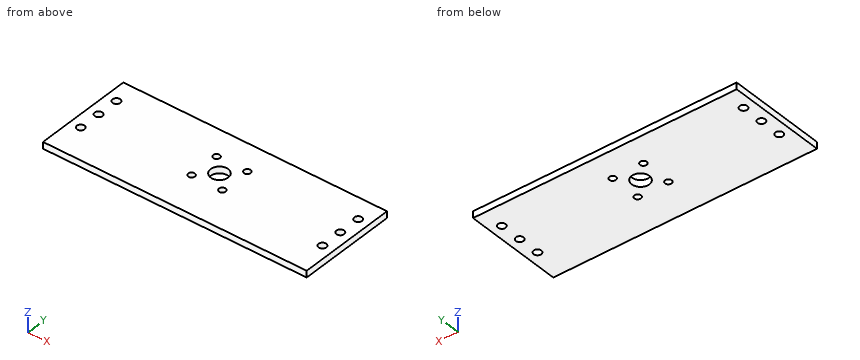
from build123d import *

# Parameters (mm, degrees)
ESQUISSE1_W             = 120
ESQUISSE1_H             = 45
BOSS_EXTRU_1_DEPTH      = 3
ESQUISSE2_R             = 1.747592995
ESQUISSE2_R_2           = 4
ESQUISSE2_R_3           = 1.5
ENL_V_MAT_EXTRU_1_DEPTH = 10


with BuildPart() as part:
    # Esquisse1 → Boss.-Extru.1 (new body)
    with BuildSketch(Plane.XY):
        Rectangle(ESQUISSE1_W, ESQUISSE1_H)
    extrude(amount=BOSS_EXTRU_1_DEPTH)

    # Esquisse2 → Enlèv. mat.-Extru.1 (cut)
    with BuildSketch(Plane.XY.offset(3)):
        with Locations((-55, 12.5)):
            Circle(ESQUISSE2_R)
        with Locations((55, 12.5)):
            Circle(ESQUISSE2_R)
        with Locations((-55, 2.5)):
            Circle(ESQUISSE2_R)
        with Locations((-55, -7.5)):
            Circle(ESQUISSE2_R)
        with Locations((55, -7.5)):
            Circle(ESQUISSE2_R)
        with Locations((55, 2.5)):
            Circle(ESQUISSE2_R)
        with Locations((0, 2.5)):
            Circle(ESQUISSE2_R_2)
        with Locations((-7, 9.5)):
            Circle(ESQUISSE2_R_3)
        with Locations((7, 9.5)):
            Circle(ESQUISSE2_R_3)
        with Locations((7, -4.5)):
            Circle(ESQUISSE2_R_3)
        with Locations((-7, -4.5)):
            Circle(ESQUISSE2_R_3)
    extrude(amount=-ENL_V_MAT_EXTRU_1_DEPTH, mode=Mode.SUBTRACT)


solid = part.part
Could you check a few things on this model? Use its own coordinates, in mm. Coordinates: 2 decimals unless noted, no trailing zeros. Write each loop counter-clockwise with the first axis right and the second up, starting at its lowest first coordinate (ties: lowest second). Pieces come first, ordered by that corner, then holes. Notation, with made-up numbers: (20.5, -12) - (33.5, -12) arc R30 cw to (33.5, 18) - close; hole circle Ø2 at (85, -33.5). An arc over 180 degrees is marked (long way). Write item = value, one per line.
1) Suppose I cut it at B-B on y = 2.5. Please give me the cut outline in (x, z), plus the area to 3 significant figures.
Result set:
outline = (-60, 0) - (-56.75, 0) - (-56.75, 3) - (-60, 3) - close; (-53.25, 0) - (-4, 0) - (-4, 3) - (-53.25, 3) - close; (4, 0) - (53.25, 0) - (53.25, 3) - (4, 3) - close; (56.75, 0) - (60, 0) - (60, 3) - (56.75, 3) - close
area = 315 mm2
2) Suppose I cut it at C-C on z = 1.6. State how many separate pieces and enclosed holes the cut face has, plus the area to 3 significant figures.
Result set:
separate_pieces = 1
enclosed_holes = 11
area = 5,260 mm2
3) Please list where these lines run through material, in increasing order: line 1 (Y direction, x = -55, z = 1.3); line 2 (Y direction, x = -7, z = 0.75); line 3 (X direction, y = 8.5, z = 1). Write a range as [from, to].
Result set:
line_1 = [-22.5, -9.25], [-5.75, 0.75], [4.25, 10.75], [14.25, 22.5]
line_2 = [-22.5, -6], [-3, 8], [11, 22.5]
line_3 = [-60, -8.12], [-5.88, 5.88], [8.12, 60]
4) Suppose I cut it at A-A on x = 0. Please give me the cut outline in (y, z).
Result set:
outline = (-22.5, 0) - (-1.5, 0) - (-1.5, 3) - (-22.5, 3) - close; (6.5, 0) - (22.5, 0) - (22.5, 3) - (6.5, 3) - close
5) Suppose I cut it at D-D on y = 12.5. Please give me the cut outline in (x, z).
Result set:
outline = (-60, 0) - (-56.75, 0) - (-56.75, 3) - (-60, 3) - close; (-53.25, 0) - (53.25, 0) - (53.25, 3) - (-53.25, 3) - close; (56.75, 0) - (60, 0) - (60, 3) - (56.75, 3) - close
6) Will this pin go through, and if not, where does the flat tip stop? pin 1 Ø2 at (x, y) = (55, 12.5) entering from +Z.
Result set:
pin_1 = through
